Can you work these out from the model? Positions are in its coordinate system, mm. Face numbers are marked on the shaded views. A direction names the side the tool comes from. Give positions to 0.01 mm unless a question says otherwise; leave off trailing zeros. Loops run counter-clockwise (first coordinate to the right, second up) from the corner with the lowest first, then second, coordinate; pieces in that order, holes last. Notation, with made-up numbers: (-39.5, 79.25) - (-7.5, 79.25) arc R29 ccw to (-7.5, 118.25) - close; hole circle Ø6 at (67.25, 21). An arc over 180 degrees is marked (long way). Write item = value, one per line.
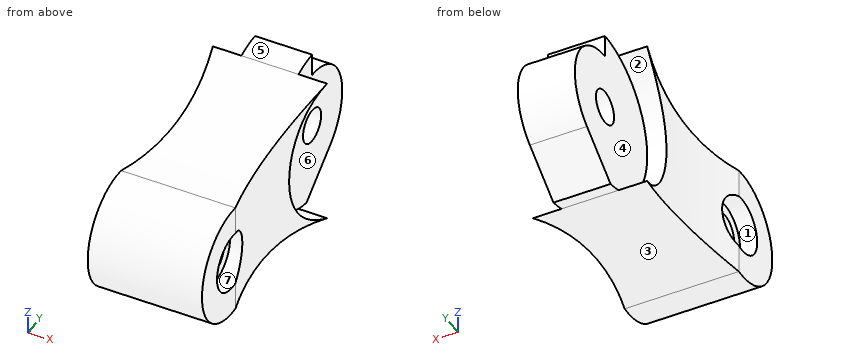
from build123d import *

# Parameters (mm, degrees)
F1_DEPTH  = 2.5
F3_DEPTH  = 5
F5_DEPTH  = 2.5
F6_R      = 7
F7_DEPTH  = 2.5
F8_R      = 7
F9_DEPTH  = 2.5
F11_DEPTH = 7.501
F12_R     = 1.5
F13_DEPTH = 10.001
F14_R     = 2.5
F15_DEPTH = 1.5
F16_R     = 2.5
F17_DEPTH = 1.5
F18_R     = 30.9477503488
F19_DEPTH = 12.5


with BuildPart() as f1:
    # F0 (on Right) → F1 (new body)
    with BuildSketch(Plane.YZ):
        with BuildLine():
            ThreePointArc((15.7492691828, 6.6282886772), (8.2400840273, 4.9647449332), (0.54884134, 4.96978603))
            ThreePointArc((0.54884134, 4.96978603), (-5, 0), (0.54884134, -4.96978603))
            ThreePointArc((0.54884134, -4.96978603), (8.2400840273, -4.9647449332), (15.7492691828, -6.6282886772))
            ThreePointArc((15.7492691828, -6.6282886772), (25, 0), (15.7492691828, 6.6282886772))
        make_face()
    extrude(amount=F1_DEPTH)

    # F2 (on face) → F3 (join)
    with BuildSketch(Plane.YZ.offset(2.5)):
        with BuildLine():
            ThreePointArc((15.7492691828, 6.6282886772), (8.2400840273, 4.9647449332), (0.54884134, 4.96978603))
            ThreePointArc((0.54884134, 4.96978603), (-5, 0), (0.54884134, -4.96978603))
            ThreePointArc((0.54884134, -4.96978603), (8.2400840273, -4.9647449332), (15.7492691828, -6.6282886772))
            ThreePointArc((15.7492691828, -6.6282886772), (25, 0), (15.7492691828, 6.6282886772))
        make_face()
    extrude(amount=F3_DEPTH)

    # F4 (on face) → F5 (join)
    with BuildSketch(Plane.YZ.offset(7.5)):
        with BuildLine():
            ThreePointArc((15.7492691828, 6.6282886772), (8.2400840273, 4.9647449332), (0.54884134, 4.96978603))
            ThreePointArc((0.54884134, 4.96978603), (-5, 0), (0.54884134, -4.96978603))
            ThreePointArc((0.54884134, -4.96978603), (8.2400840273, -4.9647449332), (15.7492691828, -6.6282886772))
            ThreePointArc((15.7492691828, -6.6282886772), (21.0150139959, -6.3174117013), (24.5686792392, -2.4191843774))
            ThreePointArc((24.5686792392, -2.4191843774), (23.0125205049, 4.8861680474), (15.7492691828, 6.6282886772))
        make_face()
    extrude(amount=F5_DEPTH)

    # F6 (on face) → F7 (cut)
    with BuildSketch(Plane.YZ.offset(10)):
        with Locations((18, 0)):
            Circle(F6_R)
    extrude(amount=-F7_DEPTH, mode=Mode.SUBTRACT)

    # F8 (on face) → F9 (cut)
    with BuildSketch(Plane(origin=(0, 0, 0), x_dir=(0, -1, 0), z_dir=(-1, 0, 0))):
        with Locations((-18, 0)):
            Circle(F8_R)
    extrude(amount=-F9_DEPTH, mode=Mode.SUBTRACT)

    # F10 (on face) → F11 (cut, through all)
    with BuildSketch(Plane.YZ.offset(7.5)):
        with BuildLine():
            ThreePointArc((18, 5), (22.7434164903, 1.5811388301), (21, -4))
            Line((21, -4), (17.0808164115, -6.9393876913))
            ThreePointArc((17.0808164115, -6.9393876913), (24.9848304861, -0.4605899264), (18, 7))
            Line((18, 7), (18, 5))
        make_face()
    extrude(amount=-F11_DEPTH, mode=Mode.SUBTRACT)

    # F12 (on face) → F13 (cut, through all)
    with BuildSketch(Plane.YZ.offset(10)):
        Circle(F12_R)
        with Locations((18, 0)):
            Circle(F12_R)
    extrude(amount=-F13_DEPTH, mode=Mode.SUBTRACT)

    # F14 (on face) → F15 (cut)
    with BuildSketch(Plane.YZ.offset(10)):
        Circle(F14_R)
    extrude(amount=-F15_DEPTH, mode=Mode.SUBTRACT)

    # F16 (on face) → F17 (cut)
    with BuildSketch(Plane(origin=(0, 0, 0), x_dir=(0, -1, 0), z_dir=(-1, 0, 0))):
        Circle(F16_R)
    extrude(amount=-F17_DEPTH, mode=Mode.SUBTRACT)

    # F18 (on Top) → F19 (cut, symmetric)
    with BuildSketch(Plane.XY):
        with Locations((-30, 8.1490552614)):
            Circle(F18_R)
        with Locations((40, 8.1490552614)):
            Circle(F18_R)
    extrude(amount=F19_DEPTH, both=True, mode=Mode.SUBTRACT)


solid = f1.part
Q1. Imagine slicing it at C-C, the plane x = 3.25. Write out the boundary of the cut face in (y, z).
Output:
outline = (0.55, -4.97) arc R35.24 cw to (15.75, -6.63) arc R7 ccw to (17.08, -6.94) - (21, -4) arc R5 ccw to (18, 5) - (18, 7) arc R7 ccw to (15.75, 6.63) arc R35.24 cw to (0.55, 4.97) arc R5 ccw (long way) to start; hole circle Ø3 at (0, 0); hole circle Ø3 at (18, 0)
Q2. Which directions (+Z, -Z, +X, -X, +Y, -Y) give clear straight access to the entire face, cutting with the end or side of a thin tool? Please do the marked faces 5, 6 and 7.
Output:
face_5 = +Z, +X, -X, -Y
face_6 = +X, +Y
face_7 = +X
Q3. Imagine slicing it at D-D, the plane y = 18.75. Write out the boundary of the cut face in (x, z).
Output:
outline = (2.5, -5.69) - (7.5, -5.69) - (7.5, -1.3) - (2.5, -1.3) - close; (2.5, 1.3) - (7.5, 1.3) - (7.5, 4.94) - (2.5, 4.94) - close
Q4. We'd pull the mould along Y, two halves only. Please class the marked faces 1, 2, 3 and 4: released by +Y, released by -Y, zero draft, split by the parting line, or undercut.
Output:
face_1 = undercut
face_2 = released by +Y
face_3 = undercut
face_4 = zero draft
Q5. Imagine slicing it at A-A, the plane y = 0. Write out the boundary of the cut face in (x, z), then the cut area to 3 significant figures.
Output:
outline = (0, -5) - (10, -5) - (10, -2.5) - (8.5, -2.5) - (8.5, -1.5) - (1.5, -1.5) - (1.5, -2.5) - (0, -2.5) - close; (0, 2.5) - (1.5, 2.5) - (1.5, 1.5) - (8.5, 1.5) - (8.5, 2.5) - (10, 2.5) - (10, 5) - (0, 5) - close
area = 64.0 mm2
Q6. For pin 1 (2 mm diameter, centred on y = 4.5, z = -4.5, fed in from -X); pin 2 (2 mm diameter, centred on x = 4.5, z = 5.5, fed in from +Y); pin 3 (1.5 mm diameter, centred on y = -1, z = -1, fed in from +X), each with a flat end and sliding along its axis, tell me the tip position at first contact or that it passes through.
Output:
pin_1 = 0.6
pin_2 = 20.18
pin_3 = 8.5
Q7. Imagine slicing it at B-B, the plane z = 1. Write out the boundary of the cut face in (x, y).
Output:
outline = (0, -4.9) - (10, -4.9) - (10, -2.29) - (8.5, -2.29) - (8.5, -1.12) - (1.5, -1.12) - (1.5, -2.29) - (0, -2.29) - close; (0.39, 2.29) - (1.5, 2.29) - (1.5, 1.12) - (8.5, 1.12) - (8.5, 2.29) - (9.61, 2.29) arc R30.95 cw to (9.19, 11.07) - (7.5, 11.07) - (7.5, 16.88) - (2.5, 16.88) - (2.5, 11.07) - (0.81, 11.07) arc R30.95 cw to start; (2.5, 19.12) - (7.5, 19.12) - (7.5, 22.9) - (2.5, 22.9) - close
Q8. I need wall thicknesses on L1, parallel to Z at x = 9.45, y = 0; L2, parallel to X at y = 20.75, z = -2.5; L3, parallel to Y at x = 9, z = 1.75. Which ranges of each line are inside material? Lowest first, please.
Output:
L1 = -5 to -2.5, 2.5 to 5
L2 = 2.5 to 7.5
L3 = -4.68 to -1.79, 1.79 to 11.22
